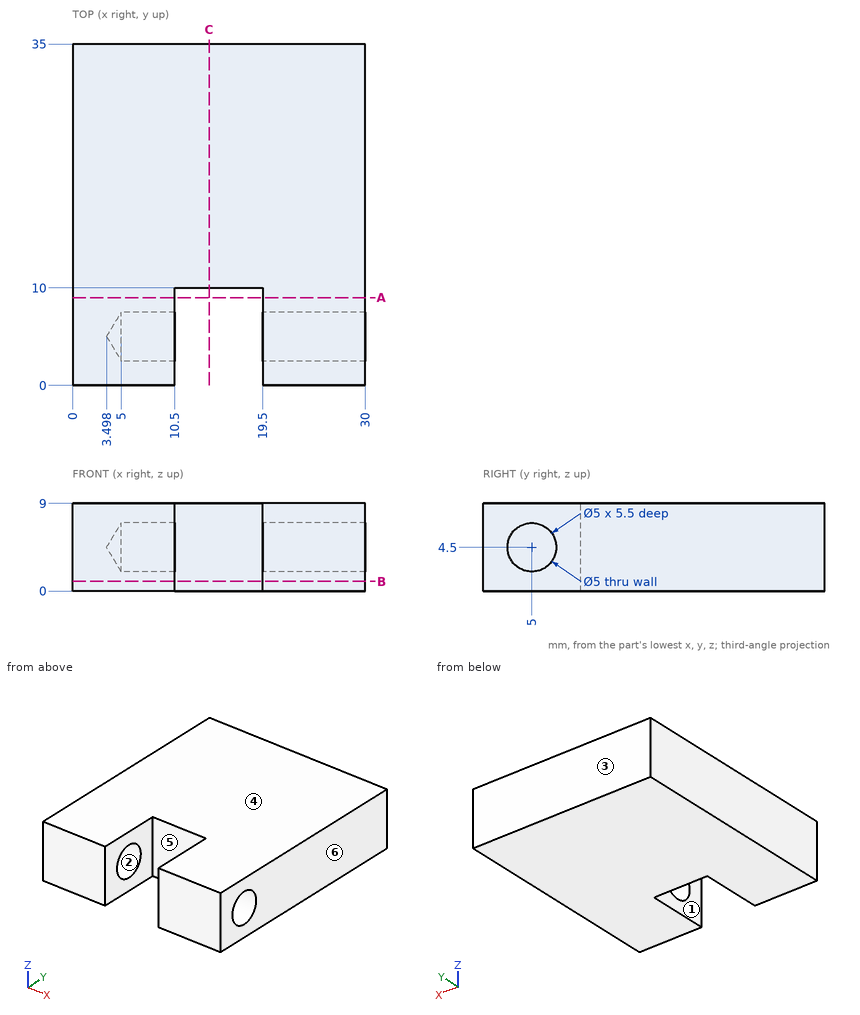
Design review of the part shown in the three views and the two pictorial views. Dimensions are in mm from the part's minimum x, y and z. A direction names the side the tool comes from. Round coordinates to 2 decimals unless told otherwise and drop trailing zeros. Write each loop counter-clockwise with the first axis right and the second up, starting at its lowest first coordinate (ties: lowest second). Pieces come first, ordered by that corner, then holes.
1) Mouldability with a two-part tool opening along X and no side actions: class the marked faces 4, 5 and 6 as +X half, -X half, draft (parallel to the pull), parting line (faces both ways), or undercut.
Answer below:
face 4: draft
face 5: undercut
face 6: +X half
2) Take a section at C-C on x = 14. Give the boundary of the cut face in (y, z).
Answer below:
outline: (10, 0) - (35, 0) - (35, 9) - (10, 9) - close
3) For line 1 along Y through (x, z) = (7, 4.5); line 2 along Z through (x, y) = (8.2, 5); line 3 along Z through (x, y) = (20.5, 4), list the stretches that pass through material, from the lowest coordinate up.
Answer below:
line 1: y = 0 to 2.5, 7.5 to 35
line 2: z = 0 to 2, 7 to 9
line 3: z = 0 to 2.21, 6.79 to 9
4) Take a section at A-A on y = 9. Give the boundary of the cut face in (x, z), then the cut area to 3 significant figures.
Answer below:
outline: (0, 0) - (10.5, 0) - (10.5, 9) - (0, 9) - close; (19.5, 0) - (30, 0) - (30, 9) - (19.5, 9) - close
area: 189 mm2
5) Take a section at B-B on z = 1. Give the boundary of the cut face in (x, y).
Answer below:
outline: (0, 0) - (10.5, 0) - (10.5, 10) - (19.5, 10) - (19.5, 0) - (30, 0) - (30, 35) - (0, 35) - close
6) Machinability: for the marked faces 1, 2 and 3, which of the approach directions +Z, -Z, +X, -X, +Y, -Y give a long, thin tool a straight path to every point of the face, cutting with its end or side? Answer none if there is none.
Answer below:
face 1: +Z, -Z, -Y
face 2: +X
face 3: +Z, -Z, +X, -X, +Y
7) Insertion check: pin 1 Ø3 at (y, z) = (5, 4.5) entering from +X. The pin has a flat end and moves straight along its axis. Give the tip position at first contact, or say it passes through.
Answer below:
pin 1: stops at x = 4.4
